```python
from build123d import *

# Parameters (mm, degrees)
F0_R     = 3
F1_DEPTH = 106
F2_DEPTH = 10
F3_DEPTH = 5
F0_W     = 3
F0_H     = 5
F4_DEPTH = 45


with BuildPart() as f1:
    # F0 (on Front) → F1 (new body)
    with BuildSketch(Plane.XZ):
        with BuildLine():
            ThreePointArc((-3.741657, -2.5), (1.306243, -4.306243), (4.5, 0))
            ThreePointArc((4.5, 0), (1.306243, 4.306243), (-3.741657, 2.5))
            ThreePointArc((-3.741657, 2.5), (-4.5, 0), (-3.741657, -2.5))
        make_face()
        Circle(F0_R, mode=Mode.SUBTRACT)
    extrude(amount=F1_DEPTH)

    # F0 (on Front) → F2 (join)
    with BuildSketch(Plane.XZ):
        Circle(F0_R)
    extrude(amount=F2_DEPTH)

    # F0 (on Front) → F3 (join)
    with BuildSketch(Plane.XZ):
        with BuildLine():
            ThreePointArc((-3.741657, -2.5), (-4.5, 0), (-3.741657, 2.5))
            Line((-3.741657, 2.5), (-7.741657, 2.5))
            Line((-7.741657, 2.5), (-7.741657, -2.5))
            Line((-7.741657, -2.5), (-3.741657, -2.5))
        make_face()
    extrude(amount=F3_DEPTH)

    # F0 (on Front) → F4 (join)
    with BuildSketch(Plane.XZ):
        with Locations((-9.241657, 0)):
            Rectangle(F0_W, F0_H)
    extrude(amount=F4_DEPTH)


solid = f1.part
```
For this review, take the finished solid that the model builds, in its own axes (mm). A direction names the side the tool comes from. Give positions to 0.01 mm unless a question says otherwise; leave off trailing zeros. Order: outer loops, then holes, each group sorted by start corner. A loop starts at its lowest first (then second) coordinate and runs counter-clockwise, first axis right, second up.
1) The part is to be moulded in two halves that separate along X. For faces 6 (the face through (-3, 0, 0)), 7 (the face through (0, -10, 0)), 8 (the face through (-10.742, -22, 0)), say which applies: released by +X, released by -X, zero draft, split by the parting line, or undercut.
2) For faces 1 (the face through (-9, -22, 2.5)), 2 (the face through (-9, -45, 0)), 3 (the face through (-7.742, -25, 0)), 4 (the face through (-9, -22, -2.5)), 5 (the face through (-3, -57, 0)), list the 3-axis set-ups (+Z, -Z, +X, -X, +Y, -Y) from which the entire face can be reached by the end or side of a thin tool; tool diameter is ignored.
3) Insertion check: pin 1 (3 mm diameter, centred on x = -8, z = 1.5, fed in from -Y); pin 2 (1 mm diameter, centred on x = -2.5, y = -45.5, fed in from +Z); pin 3 (4 mm diameter, centred on y = -63, z = -0.5, fed in from -X). Each pin has a flat end and moves straight along its axis. Give the tip position at first contact, or say it passes through.
4) Wall thickness on line 1 (Z direction, x = 0, y = -32); line 2 (X direction, y = -14, z = -0.75); line 3 (Y direction, x = -0.75, z = 1.75): over which ranges is each line inside the solid? List them lowest first.
5) Take a section at B-B (x = 0). Give the boundary of the cut face in (y, z), then the cut area to 3 significant figures.
6) Take a section at D-D (y = -85). Give the boundary of the cut face in (x, z).
7) Take a section at C-C (z = -1.25). Give the boundary of the cut face in (x, y), then the cut area to 3 significant figures.
8) Take a section at A-A (y = -11.5). Give the boundary of the cut face in (x, z).
Derived:
1. face 6: zero draft
1. face 7: undercut
1. face 8: released by -X
2. face 1: +Z, -X, +Y, -Y
2. face 2: +Z, -Z, -X, -Y
2. face 3: +Z, -Z, -Y
2. face 4: -Z, -X, +Y, -Y
2. face 5: -Y
3. pin 1: stops at y = -45
3. pin 2: stops at z = 4.03
3. pin 3: stops at x = -4.5
4. line 1: z = -4.5 to -3, 3 to 4.5
4. line 2: x = -10.74 to -7.74, -4.44 to -2.9, 2.9 to 4.44
4. line 3: y = -10 to 0
5. outline: (-106, -4.5) - (0, -4.5) - (0, 4.5) - (-106, 4.5) - (-106, 3) - (-10, 3) - (-10, -3) - (-106, -3) - close
5. area: 378 mm2
6. outline: (-3.74, -2.5) arc R4.5 ccw (long way) to (-3.74, 2.5) arc R4.5 ccw to start; hole circle Ø6 at (0, 0)
7. outline: (-10.74, -45) - (-7.74, -45) - (-7.74, -5) - (-4.32, -5) - (-4.32, -106) - (-2.73, -106) - (-2.73, -10) - (2.73, -10) - (2.73, -106) - (4.32, -106) - (4.32, 0) - (-10.74, 0) - close
7. area: 545 mm2
8. outline: (-10.74, -2.5) - (-7.74, -2.5) - (-7.74, 2.5) - (-10.74, 2.5) - close; (-3.74, -2.5) arc R4.5 ccw (long way) to (-3.74, 2.5) arc R4.5 ccw to start; hole circle Ø6 at (0, 0)
